from build123d import *

# Parameters (mm, degrees)
SKETCH1_R           = 7.6
SKETCH1_R_2         = 2.25
BOSS_EXTRUDE1_DEPTH = 24
BOSS_EXTRUDE2_DEPTH = 19.25
CUT_EXTRUDE1_DEPTH  = 56.448737587
CHAMFER1_SIZE       = 6
SKETCH6_R           = 2.25
CUT_EXTRUDE3_DEPTH  = 16
CHAMFER2_SIZE       = 6


with BuildPart() as part:
    # Sketch1 → Boss-Extrude1 (new body)
    with BuildSketch(Plane(origin=(0, 0, 0), x_dir=(1, 0, 0), z_dir=(0, 1, 0))):
        with BuildLine():
            Line((-9.625, -8.5), (9.625, -8.5))
            Line((9.625, -8.5), (9.625, 0))
            ThreePointArc((9.625, 0), (9.506941676, 1.502892202), (9.155662863, 2.968916054))
            Line((9.155662863, 2.968916054), (4.796712187, 16.411223653))
            ThreePointArc((4.796712187, 16.411223653), (0, 20), (-4.796712187, 16.411223653))
            Line((-4.796712187, 16.411223653), (-9.155662863, 2.968916054))
            ThreePointArc((-9.155662863, 2.968916054), (-9.506941676, 1.502892202), (-9.625, 0))
            Line((-9.625, 0), (-9.625, -8.5))
        make_face()
        with Locations(Location((0, 0, 0), (0, 0, 270))):
            Circle(SKETCH1_R, mode=Mode.SUBTRACT)
        with Locations(Location((0, 15, 0), (0, 0, 270))):
            Circle(SKETCH1_R_2, mode=Mode.SUBTRACT)
    extrude(amount=BOSS_EXTRUDE1_DEPTH)

    # Sketch3 → Boss-Extrude2 (add)
    with BuildSketch(Plane.ZY.offset(9.625)):
        Polygon((8.5, 0), (14.5, 0), (14.5, 48), (8.5, 48), (8.5, 24), align=None)
    extrude(amount=-BOSS_EXTRUDE2_DEPTH)

    # Sketch4 → Cut-Extrude1 (cut, through all)
    with BuildSketch(Plane(origin=(9.625, 0, 0), x_dir=(0, 0, -1), z_dir=(1, 0, 0))):
        Polygon((-14.5, 0), (-14.5, 6), (-3.5, 0), align=None)
    extrude(amount=-CUT_EXTRUDE1_DEPTH, mode=Mode.SUBTRACT)

    # Chamfer1
    chamfer1_edges = [part.edges().sort_by_distance(p)[0] for p in [
        (-9.625, 48, 11.5),
    ]]
    chamfer(chamfer1_edges, length=CHAMFER1_SIZE)

    # Sketch6 → Cut-Extrude3 (cut)
    with BuildSketch(Plane.XY.offset(14.5)):
        with Locations((0, 14.504303095)):
            Circle(SKETCH6_R)
        with Locations((0, 31.5)):
            Circle(SKETCH6_R)
    extrude(amount=-CUT_EXTRUDE3_DEPTH, mode=Mode.SUBTRACT)

    # Chamfer2
    chamfer2_edges = [part.edges().sort_by_distance(p)[0] for p in [
        (3, 48, 8.5),
    ]]
    chamfer(chamfer2_edges, length=CHAMFER2_SIZE - 0.0001)  # a hair under: the kernel refuses the full size


solid = part.part
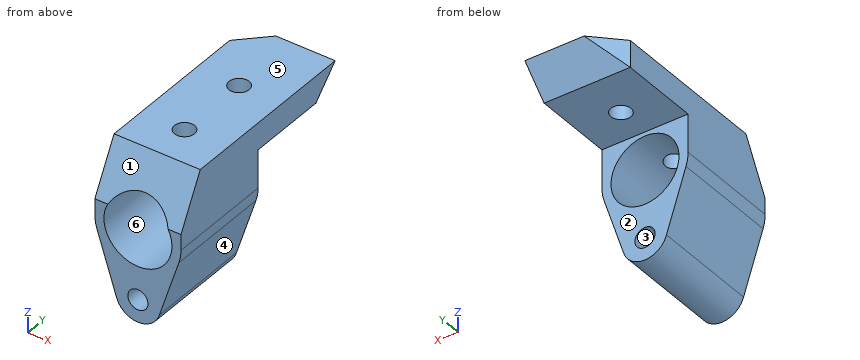
Read the model definition and answer for the solid it produces. Units are mm, in the model's axes. Face numbers are marked on the shaded views. A direction names the side the tool comes from. Coordinates: 2 decimals unless noted, no trailing zeros. Loops run counter-clockwise (first coordinate to the right, second up) from the corner with the lowest first, then second, coordinate; pieces in that order, holes last.
Q1. Each of these flat-tipped pins is pushed along its axis until it touches: pin 1 Ø6 at (x, z) = (3, -7) entering from +Y; pin 2 Ø6 at (y, z) = (29.5, -14.5) entering from -X; pin 3 Ø8 at (x, z) = (-5, 5.5) entering from +Y; pin 4 Ø3.5 at (x, y) = (0, 14.5) entering from +Z. Where does it stop, or does it pass through?
Q2. Consider probe 1 along Z at (x, y) = (-1.75, 22); probe 2 along Y at (x, z) = (0, 10.25); probe 3 along X at (y, z) = (8.25, 0) (3 decimals). Determine where each line is inside the solid, lowest interval first.
Q3. The part is cut by section B-B on z = -4. Write down the section's boundary in (x, y).
Q4. Which of the six approach directions +Z, -Z, +X, -X, +Y, -Y give full straight-line access (tool end or side, diameter ignored) to the marked faces 1 and 2?
Q5. The mould has two halves that part along X. Classify the marked faces 3, 4, 5 and 6: +X half, -X half, draft (parallel to the pull), parting line (faces both ways), or undercut.
Q6. The part is cut by section A-A on y = 31.5. Write down the section's boundary in (x, z) (3 decimals), and give its area (3 significant figures).
Q7. The part is cut by section D-D on x = 0. Give the number of separate pieces and of enclosed holes in the cut face, and give its area (3 significant figures).
Results below:
1. pin 1: stops at y = 24
1. pin 2: passes through
1. pin 3: stops at y = 43
1. pin 4: stops at z = -7.4
2. probe 1: z = -19.68 to -16.41, -13.59 to -7.4, 7.4 to 14.5
2. probe 2: y = 3.68 to 12.25, 16.75 to 29.25, 33.75 to 43.75
2. probe 3: x = -9.625 to -7.6, 7.6 to 9.625
3. outline: (-8.82, 0) - (-6.46, 0) - (-6.46, 24) - (-8.82, 24) - close; (6.46, 0) - (8.82, 0) - (8.82, 24) - (6.46, 24) - close
4. face 1: +Z, +X, -X, -Y
4. face 2: -Z, +X, -X, +Y
5. face 3: undercut
5. face 4: +X half
5. face 5: draft
5. face 6: undercut
6. outline: (-9.625, 8.5) - (-2.25, 8.5) - (-2.25, 14.5) - (-9.625, 14.5) - close; (2.25, 8.5) - (9.625, 8.5) - (9.625, 14.5) - (2.25, 14.5) - close
6. area: 88.5 mm2
7. separate pieces: 5
7. enclosed holes: 0
7. area: 395 mm2
